Verification items for this drawing (mm, ordinates from the low corner). A direction names the side the tool comes from. Round coordinates to 2 decimals unless told otherwise and drop trailing zeros. Order: outer loops, then holes, each group sorted by start corner. A loop starts at its lowest first (then second) coordinate and runs counter-clockwise, first axis right, second up.
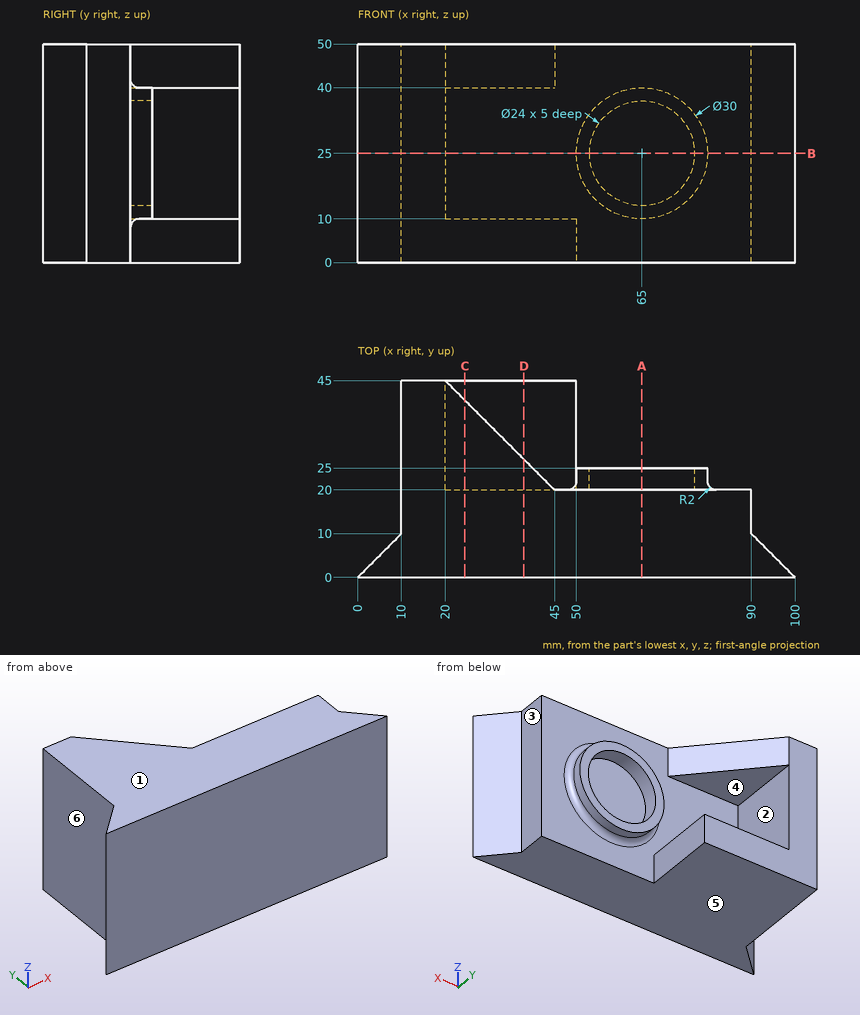
Item 1: Release check for a two-part mould opening along Z. For the marked faces 4, 5 and 6 record: released by +Z, released by -Z, zero draft, split by the parting line, or undercut.
Answer:
face 4: undercut
face 5: released by -Z
face 6: zero draft
Item 2: Scan lines: line 1 along Z through (x, y) = (65, 23.1); line 2 along Z through (x, y) = (22, 21.5); line 3 along Y through (x, z) = (45, 40). Record each from-to range of solid material in increasing order.
Answer:
line 1: z = 10 to 13, 37 to 40
line 2: z = 0 to 10, 40 to 50
line 3: y = 0 to 20
Item 3: Go/stop test with flat-tipped pins: P1, Ø5, axis at y = 35, z = 3.5, coming from the +X side; P2, Ø7.5, axis at y = 36.5, z = 25.5, coming from the +X side; P3, Ø24, axis at x = 62, z = 18.5, coming from the +Y side. Record where each tip stops, or that it passes through.
Answer:
P1: stops at x = 50
P2: stops at x = 20
P3: stops at y = 25
Item 4: Access from +Z, -Z, +X, -X, +Y, -Y to the whole of each face (thin tool, end or side, straight path). Record for the marked faces 1, 2 and 3.
Answer:
face 1: +Z, +X, -X, +Y, -Y
face 2: +Y
face 3: +Z, -Z, +X, +Y
Item 5: Sectioned sample at A-A (x = 65). Record the cut outline in (y, z), and give its area (3 significant figures).
Answer:
outline: (0, 0) - (20, 0) - (20, 8) arc R2 cw to (22, 10) - (25, 10) - (25, 13) - (20, 13) - (20, 37) - (25, 37) - (25, 40) - (22, 40) arc R2 cw to (20, 42) - (20, 50) - (0, 50) - close
area: 1,030 mm2
Item 6: Sectioned sample at B-B (z = 25). Record the cut outline in (x, y).
Answer:
outline: (0, 0) - (100, 0) - (90, 10) - (90, 20) - (82, 20) arc R2 cw to (80, 22) - (80, 25) - (77, 25) - (77, 20) - (53, 20) - (53, 25) - (50, 25) - (50, 22) arc R2 cw to (48, 20) - (20, 20) - (20, 45) - (10, 45) - (10, 10) - close
Item 7: Sectioned sample at D-D (x = 38). Record the cut outline in (y, z).
Answer:
outline: (0, 0) - (45, 0) - (45, 10) - (20, 10) - (20, 40) - (27, 40) - (27, 50) - (0, 50) - close
Item 8: Sectioned sample at C-C (x = 24.5). Record the cut outline in (y, z).
Answer:
outline: (0, 0) - (45, 0) - (45, 10) - (20, 10) - (20, 40) - (40.5, 40) - (40.5, 50) - (0, 50) - close
